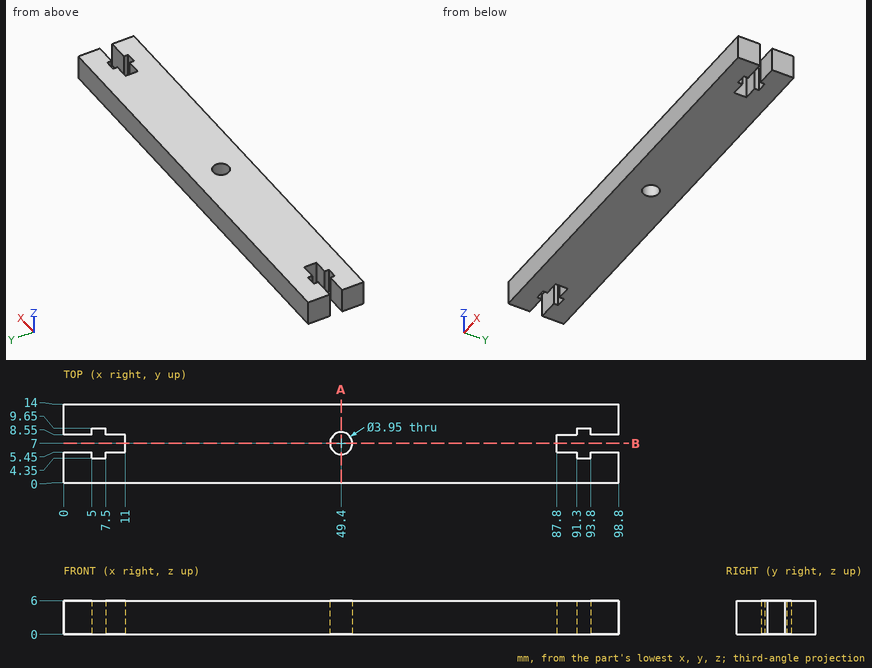
Input: dimensioned drawing with shaded views. Units: mm. Origin: part minimum x, y, z. Round coordinates to 2 decimals unless told otherwise and drop trailing zeros. Loops run counter-clockwise (first coordinate to the right, second up) from the corner with the lowest first, then second, coordinate; pieces in that order, holes last. Notation, with made-up numbers: M -38.5,28.5 L -0.5,28.5 A26 cw -0.5,58.5 Z; hole C 46,-31.5 d1. An arc over 180 degrees is marked long. Return JSON: item names as keys, results as strings. Group by question number.
1. Section query B-B on y = 7. Output: boundary loops of the cut face in (x, z) (3 decimals), and give its area (3 significant figures).
2. Material intervals for line 1 along Y through (x, z) = (49.4, 2) (3 decimals); line 2 along Y through (x, z) = (90.5, 1.6), sorted ascending. Write a range as from..to.
3. Pin query (flat end, axial travel): pin 1 (0.9 mm diameter, centred on y = 7, z = 4.5, fed in from -X); pin 2 (0.9 mm diameter, centred on y = 6.5, z = 4, fed in from +X). Return the tip coordinate at first contact, or that it passes through.
4. Section query A-A on x = 49.4. Output: boundary loops of the cut face in (y, z) (3 decimals).
Checks:
{
 "1": {"outline": "M 11,0 L 47.425,0 L 47.425,6 L 11,6 Z; M 51.375,0 L 87.8,0 L 87.8,6 L 51.375,6 Z", "area": "437 mm²"},
 "2": {"line 1": "y = 0..5.025, 8.975..14", "line 2": "y = 0..5.45, 8.55..14"},
 "3": {"pin 1": "stops at x = 11", "pin 2": "stops at x = 87.8"},
 "4": {"outline": "M 0,0 L 5.025,0 L 5.025,6 L 0,6 Z; M 8.975,0 L 14,0 L 14,6 L 8.975,6 Z"}
}
